from build123d import *

# Parameters (mm, degrees)
SKETCH_1_W          = 600
SKETCH_1_H          = 600
EXTRUDE_1_DEPTH     = 20
SKETCH_2_W          = 100
SKETCH_2_H          = 100
EXTRUDE_2_DEPTH     = 20
SKETCH_3_R          = 20
EXTRUDE_3_DEPTH     = 5
EXTRUDE_START       = -5
SKETCH_5_R          = 20
EXTRUDE_4_DEPTH     = 5
EXTRUDE_1_2_DEPTH   = 15
SKETCH_7_R          = 25
CUT_EXTRUDE_1_DEPTH = 20


with BuildPart() as part:
    # 草图1 → Extrude 1 (new body)
    with BuildSketch(Plane(origin=(0, 0, 0), x_dir=(1, 0, 0), z_dir=(0, 1, 0))):
        Rectangle(SKETCH_1_W, SKETCH_1_H)
    extrude(amount=EXTRUDE_1_DEPTH)

    # 草图2 → 凸台-拉伸2 (add)
    with BuildSketch(Plane(origin=(0, 20, 0), x_dir=(1, 0, 0), z_dir=(0, 1, 0))):
        with Locations((205.348971612, -11.468548329)):
            Rectangle(SKETCH_2_W, SKETCH_2_H)
    extrude(amount=EXTRUDE_2_DEPTH)

    # 草图3 → 凸台-拉伸3 (add)
    with BuildSketch(Plane.XY.offset(61.468548329)):
        with BuildLine():
            Line((255.348971612, 40), (255.348971612, 114.766543298))
            ThreePointArc((255.348971612, 114.766543298), (205.348971612, 164.766543298), (155.348971612, 114.766543298))
            Line((155.348971612, 114.766543298), (155.348971612, 40))
            Line((155.348971612, 40), (255.348971612, 40))
        make_face()
        with Locations((205.348971612, 114.766543298)):
            Circle(SKETCH_3_R, mode=Mode.SUBTRACT)
    extrude(amount=-EXTRUDE_3_DEPTH)

    # 草图5 → 凸台-拉伸4 (add)
    with BuildSketch(Plane(origin=(0, 0, -38.531451671), x_dir=(-1, 0, 0), z_dir=(0, 0, -1)).offset(EXTRUDE_START)):
        with BuildLine():
            ThreePointArc((-255.348971612, 114.766543298), (-205.348971612, 164.766543298), (-155.348971612, 114.766543298))
            Line((-155.348971612, 114.766543298), (-155.348971612, 40))
            Line((-155.348971612, 40), (-255.348971612, 40))
            Line((-255.348971612, 40), (-255.348971612, 114.766543298))
        make_face()
        with Locations(Location((-205.348971612, 114.766543298, 0), (0, 0, 180))):
            Circle(SKETCH_5_R, mode=Mode.SUBTRACT)
    extrude(amount=EXTRUDE_4_DEPTH)

    # 草图6 → Extrude 1 2 (add)
    with BuildSketch(Plane(origin=(0, 20, 0), x_dir=(1, 0, 0), z_dir=(0, 1, 0))):
        with BuildLine():
            Line((-194.645221659, -69.468548329), (85.354778341, -69.468548329))
            ThreePointArc((85.354778341, -69.468548329), (116.854778341, -100.968548329), (85.354778341, -132.468548329))
            Line((85.354778341, -132.468548329), (-194.645221659, -132.468548329))
            ThreePointArc((-194.645221659, -132.468548329), (-226.145221659, -100.968548329), (-194.645221659, -69.468548329))
        make_face()
        with BuildLine():
            Line((-194.645221659, -71.468548329), (85.354778341, -71.468548329))
            ThreePointArc((85.354778341, -71.468548329), (114.854778341, -100.968548329), (85.354778341, -130.468548329))
            Line((85.354778341, -130.468548329), (-194.645221659, -130.468548329))
            ThreePointArc((-194.645221659, -130.468548329), (-224.145221659, -100.968548329), (-194.645221659, -71.468548329))
        make_face(mode=Mode.SUBTRACT)
    extrude(amount=EXTRUDE_1_2_DEPTH)

    # 草图7 → 切除-拉伸1 (cut)
    with BuildSketch(Plane(origin=(0, 20, 0), x_dir=(1, 0, 0), z_dir=(0, 1, 0))):
        with Locations(Location((0, 0, 0), (0, 0, 270))):
            Circle(SKETCH_7_R)
    extrude(amount=-CUT_EXTRUDE_1_DEPTH, mode=Mode.SUBTRACT)


solid = part.part
Could you check a few things on this model? Use its own coordinates, in mm. A direction names the side the tool comes from. Give positions to 0.01 mm unless a question says otherwise; leave off trailing zeros. Write each loop counter-clockwise with the first axis right and the second up, starting at its lowest first coordinate (ties: lowest second). Pieces come first, ordered by that corner, then holes. Notation, with made-up numbers: (-20, 43.5) -> (5, 43.5) arc R6 ccw to (5, 48.5) -> close; hole circle Ø1 at (40.25, 65). An arc over 180 degrees is marked (long way). Answer as CSV lines item,"result". Start each with the question number.
(1) Please list where these lines run through material, in increasing order: line 1 (X direction, y = 9.25, z = 0); line 2 (Z direction, x = 57, y = 22); line 3 (Y direction, x = -75.5, z = -17).
(2) I'm going to push flat-ended pins straight in: pin 1 Ø4 at (x, z) = (-151.5, -162.5) entering from +Y; pin 2 Ø8 at (y, z) = (27, 169.5) entering from -X; pin 3 Ø16.5 at (x, y) = (-30.5, 29.5) entering from +Z; pin 4 Ø10 at (x, y) = (238, 142) entering from -Z. Where does each tip first touch, or does it pass through?
(3) If we mould it in two halves opening along X, with no side actions, what happens to faces 4 (the face through (-224.14, 27.4, 101.62)), 5 (the face through (300, 10, 4)), 6 (the face through (205, 93, -38.531)), 7 (the face through (7.509, 10.14, 23.846))? For each: +X half, -X half, draft (parallel to the pull), parting line (faces both ways), or undercut.
(4) If we section it at B-B, the plane x = 0: Write out the boundary of the cut face in (y, z).
(5) If we section it at A-A, the plane y = 70: Write out the boundary of the cut face in (x, z).
(6) Which directions (+Z, -Z, +X, -X, +Y, -Y) give clear straight access to the entire face, cutting with the end or side of a thin tool? Please do faces 1 (the face through (-57, 27, 71.469)), 2 (the face through (116.847, 27.395, 100.276)), 3 (the face through (205, 89, 56.469)).
(7) If we section it at C-C, the plane z = 0: Write out the boundary of the cut face in (x, y).
(8) If we section it at D-D, the plane y = 124: Write out the boundary of the cut face in (x, z).
Answer list:
1,line 1,"-300 to -25, 25 to 300"
1,line 2,"69.47 to 71.47, 130.47 to 132.47"
1,line 3,"0 to 20"
2,pin 1,"y = 20"
2,pin 2,"through"
2,pin 3,"z = 132.47"
2,pin 4,"z = -38.53"
3,face 4,"undercut"
3,face 5,"+X half"
3,face 6,"draft"
3,face 7,"undercut"
4,outline,"(0, -300) -> (20, -300) -> (20, -25) -> (0, -25) -> close; (0, 25) -> (20, 25) -> (20, 69.47) -> (35, 69.47) -> (35, 71.47) -> (20, 71.47) -> (20, 130.47) -> (35, 130.47) -> (35, 132.47) -> (20, 132.47) -> (20, 300) -> (0, 300) -> close"
5,outline,"(155.35, -38.53) -> (255.35, -38.53) -> (255.35, -33.53) -> (155.35, -33.53) -> close; (155.35, 56.47) -> (255.35, 56.47) -> (255.35, 61.47) -> (155.35, 61.47) -> close"
6,face 1,"+Y"
6,face 2,"+X, +Y"
6,face 3,"+X, -X, +Y"
7,outline,"(-300, 0) -> (-25, 0) -> (-25, 20) -> (-300, 20) -> close; (25, 0) -> (300, 0) -> (300, 20) -> (255.35, 20) -> (255.35, 40) -> (155.35, 40) -> (155.35, 20) -> (25, 20) -> close"
8,outline,"(156.21, -38.53) -> (187.61, -38.53) -> (187.61, -33.53) -> (156.21, -33.53) -> close; (156.21, 56.47) -> (187.61, 56.47) -> (187.61, 61.47) -> (156.21, 61.47) -> close; (223.09, -38.53) -> (254.49, -38.53) -> (254.49, -33.53) -> (223.09, -33.53) -> close; (223.09, 56.47) -> (254.49, 56.47) -> (254.49, 61.47) -> (223.09, 61.47) -> close"
